The model under review builds one solid part; all positions refer to its coordinate system, in mm. Face numbers are marked on the shaded views. A direction names the side the tool comes from. Give positions to 0.01 mm unless a question says otherwise; leave off trailing zeros. Order: outer loops, then holes, each group sorted by start corner. A loop starts at its lowest first (then second) coordinate and runs counter-clockwise, first axis right, second up.
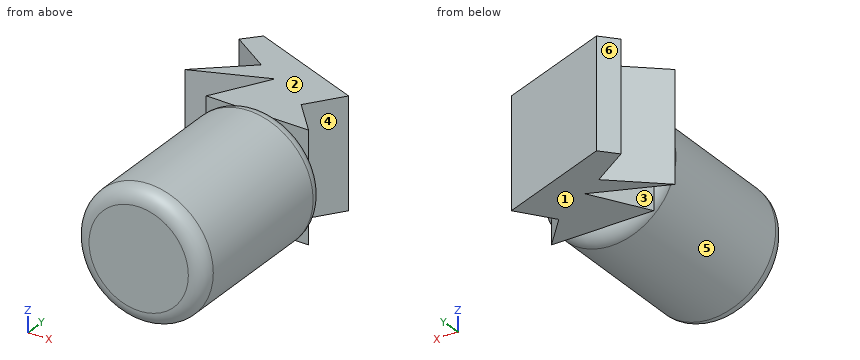
```python
from build123d import *

# Parameters (mm, degrees)
F0_R     = 21.993212
F1_DEPTH = 60.56268
F2_R     = 5.08
F4_DEPTH = 18.65978


with BuildPart() as f1:
    # F0 (on Front) → F1 (new body)
    with BuildSketch(Plane.XZ):
        Circle(F0_R)
    extrude(amount=F1_DEPTH)

    # F2
    f2_edges = [f1.edges().sort_by_distance(p)[0] for p in [
        (21.993212, -30.28134, 0),
        (-21.993212, 0, 0),
        (-21.993212, -60.56268, 0),
    ]]
    fillet(f2_edges, radius=F2_R)

    # F3 (on Top) → F4 (join, symmetric)
    with BuildSketch(Plane.XY):
        Polygon((-17.87933, 0), (16.99487, 0), (7.151732, 10.876591), (15.49542, 22.498155), (-23.541117, 37.397597), (-28.308937, 32.033801), (-14.899442, 23.392122), (-31.288829, 9.08866), (-7.151735, 18.922292), align=None)
    extrude(amount=F4_DEPTH, both=True)


solid = f1.part
```
1. Take a section at D-D (y = -8.5). Write out the cut boundary in (x, z), and give its area (3 significant figures).
2. Take a section at C-C (x = 0). Write out the cut boundary in (y, z), and give its area (3 significant figures).
3. To check wall thickness, follow line 1 (Y direction, x = -7.5, z = -18); line 2 (Z direction, x = -11, y = 29.5); line 3 (Y direction, x = 7.5, z = 5). State the ranges of each line that lie inside material, in increasing order.
4. Take a section at B-B (z = 0). Write out the cut boundary in (x, y).
5. Insertion check: pin 1 (4 mm diameter, centred on x = -3.5, y = -31, fed in from -Z); pin 2 (1 mm diameter, centred on x = -20, z = 7.5, fed in from +Y); pin 3 (8 mm diameter, centred on x = -10, y = -42, fed in from -Z). Each pin has a flat end and moves straight along its axis. Give the tip position at first contact, or say it passes through.
6. Draft analysis for pull direction Y (two halves, no side actions). For the marked faces 4, 5 and 6, state which applies: pulls with the +Y half, pulls with the -Y half, needs draft (parallel to the pull), parting line crosses it, or undercut.
7. Take a section at A-A (y = 16.5). Write out the cut boundary in (x, z) (3 decimals), and give its area (3 significant figures).
8. For the marked faces 1, 2 and 3, list the 3-axis set-ups (+Z, -Z, +X, -X, +Y, -Y) from which the entire face can be reached by the end or side of a thin tool; tool diameter is ignored.
Answer:
1. outline: circle Ø43.99 at (0, 0)
1. area: 1,520 mm2
2. outline: (-60.56, -16.91) arc R5.08 ccw to (-55.48, -21.99) - (-5.08, -21.99) arc R5.08 ccw to (0, -16.91) - (0, -18.66) - (28.41, -18.66) - (28.41, 18.66) - (0, 18.66) - (0, 16.91) arc R5.08 ccw to (-5.08, 21.99) - (-55.48, 21.99) arc R5.08 ccw to (-60.56, 16.91) - close
2. area: 3,700 mm2
3. line 1: y = -59.85 to -0.71, 0 to 18.31, 18.78 to 31.28
3. line 2: z = -18.66 to 18.66
3. line 3: y = -60.56 to 10.49, 11.36 to 25.55
4. outline: (-31.29, 9.09) - (-7.15, 18.92) - (-17.88, 0) - (-16.91, 0) arc R5.08 ccw to (-21.99, -5.08) - (-21.99, -55.48) arc R5.08 ccw to (-16.91, -60.56) - (16.91, -60.56) arc R5.08 ccw to (21.99, -55.48) - (21.99, -5.08) arc R5.08 ccw to (16.91, 0) - (16.99, 0) - (7.15, 10.88) - (15.5, 22.5) - (-23.54, 37.4) - (-28.31, 32.03) - (-14.9, 23.39) - close
5. pin 1: stops at z = -21.94
5. pin 2: stops at y = 36.24
5. pin 3: stops at z = -21.16
6. face 4: undercut
6. face 5: needs draft
6. face 6: pulls with the +Y half
7. outline: (-22.797, -18.66) - (-13.097, -18.66) - (-13.097, 18.66) - (-22.797, 18.66) - close; (-8.525, -18.66) - (11.189, -18.66) - (11.189, 18.66) - (-8.525, 18.66) - close
7. area: 1,100 mm2
8. face 1: -Z, +X, -X, +Y
8. face 2: +Z, +X, -X, +Y
8. face 3: +Z, -Z
